from build123d import *

# Parameters (mm, degrees)
SKETCH2_W               = 9.652
SKETCH2_H               = 3.048
SKETCH2_W_2             = 3.048
SKETCH2_H_2             = 35.052
BOSS_EXTRUDE1_DEPTH     = 315
SKETCH3_W               = 25.4
SKETCH3_H               = 76.2
SKETCH3_W_2             = 19.304
SKETCH3_H_2             = 70.104
BOSS_EXTRUDE2_DEPTH     = 50
CUT_EXTRUDE1_DEPTH      = 1
CUT_EXTRUDE1_DEPTH_BACK = 77.2


with BuildPart() as part:
    # Sketch2 → Boss-Extrude1 (new body)
    with BuildSketch(Plane.XY):
        Polygon((-12.7, 0), (-9.652, 0), (-9.652, 35.052), (-9.652, 38.1), (-12.7, 38.1), align=None)
        with Locations((-4.826, 36.576)):
            Rectangle(SKETCH2_W, SKETCH2_H)
        Polygon((0, 38.1), (0, 35.052), (9.652, 35.052), (9.652, 0), (12.7, 0), (12.7, 38.1), align=None)
        with Locations((11.176, -17.526)):
            Rectangle(SKETCH2_W_2, SKETCH2_H_2)
        Polygon((-9.652, -35.052), (-9.652, 0), (-12.7, 0), (-12.7, -38.1), (0, -38.1), (0, -35.052), align=None)
        Polygon((9.652, -35.052), (0, -35.052), (0, -38.1), (12.7, -38.1), (12.7, -35.052), align=None)
    extrude(amount=BOSS_EXTRUDE1_DEPTH)

    # Sketch3 → Boss-Extrude2 (add)
    with BuildSketch(Plane(origin=(0, 0, 0), x_dir=(-1, 0, 0), z_dir=(0, 0, -1))):
        Rectangle(SKETCH3_W, SKETCH3_H)
        Rectangle(SKETCH3_W_2, SKETCH3_H_2, mode=Mode.SUBTRACT)
    extrude(amount=BOSS_EXTRUDE2_DEPTH)

    # Sketch4 → Cut-Extrude1 (cut, two sides)
    with BuildSketch(Plane(origin=(0, 38.1, 0), x_dir=(1, 0, 0), z_dir=(0, 1, 0))) as cut_extrude1_sk:
        Polygon((12.7, 48.301505629), (115.189557491, -14.672106721), (124.098071564, 55.267937569), (-106.281043419, 84.612151011), (-115.189557491, 14.672106721), (-12.7, 1.617644511), (-12.7, 50), (12.7, 50), align=None)
        Polygon((12.7, -1.617644511), (115.189557491, -14.672106721), (12.7, 48.301505629), align=None)
        Polygon((0, 0), (12.7, -1.617644511), (12.7, 48.301505629), (12.534006261, 48.403498707), align=None)
        Polygon((12.534006261, 48.403498707), (12.7, 48.301505629), (12.7, 50), (-12.7, 50), (-12.7, 1.617644511), (0, 0), align=None)
    extrude(amount=CUT_EXTRUDE1_DEPTH, mode=Mode.SUBTRACT)
    extrude(cut_extrude1_sk.sketch, amount=-CUT_EXTRUDE1_DEPTH_BACK, mode=Mode.SUBTRACT)


solid = part.part
Geometry: final body of the model. Coordinates: model frame, mm. A direction names the side the tool comes from. Give positions to 0.01 mm unless a question says otherwise; leave off trailing zeros. Write each loop counter-clockwise with the first axis right and the second up, starting at its lowest first coordinate (ties: lowest second). Pieces come first, ordered by that corner, then holes. Notation, with made-up numbers: (-11, 16) -> (36, 16) arc R23 cw to (36, 47) -> close; hole circle Ø5 at (-25.5, 51.5). An arc over 180 degrees is marked (long way). Answer in a Markdown table with one row per item.
(1) Section query C-C on x = -5.75. Return loops of the section in (y, z), then the cut area to 3 significant figures.
Answers below:
| item | result |
|---|---|
| outline | (-38.1, -0.73) -> (-35.05, -0.73) -> (-35.05, 315) -> (-38.1, 315) -> close; (35.05, -0.73) -> (38.1, -0.73) -> (38.1, 315) -> (35.05, 315) -> close |
| area | 1,920 mm^2 |
(2) Draft query along X for faces 3 (the flat face through (9.652, 0, 160)), 4 (the flat face through (0, 35.052, 159)), 5 (the flat face through (-10, 3, 315)), 6 (the flat face through (-10.407, 3, -1.326)). Return one class per face: +X half, -X half, draft (parallel to the pull), parting line (faces both ways), or undercut.
Answers below:
| item | result |
|---|---|
| face 3 | undercut |
| face 4 | undercut |
| face 5 | draft |
| face 6 | +X half |
(3) Ray query, line 1 along X through (y, z) = (-2, 140.5); line 2 along Y through (x, z) = (4.5, 220); line 3 along Z through (x, y) = (11.25, -10). Return the intervals inside material, ascending. Write a range as [from, to].
Answers below:
| item | result |
|---|---|
| line 1 | [-12.7, -9.65], [9.65, 12.7] |
| line 2 | [-38.1, -35.05], [35.05, 38.1] |
| line 3 | [1.43, 315] |
(4) Set-up query: faces 1 (the flat face through (12.7, -1, 161)), 2 (the flat face through (-9.652, 0, 159)). Return all of +Z, -Z, +X, -X, +Y, -Y with unobstructed straight access to the full face (end or side cutting, diameter ignored); none if empty.
Answers below:
| item | result |
|---|---|
| face 1 | +Z, -Z, +X, +Y, -Y |
| face 2 | +Z, -Z |
(5) Pin query (flat end, axial travel): pin 1 (8 mm diameter, centred on x = 9, y = 7.5, fed in from +Z). Return the tip coordinate at first contact, or that it passes through.
Answers below:
| item | result |
|---|---|
| pin 1 | z = 315 |
(6) Section query B-B on z = 54. Return loops of the section in (x, y).
Answers below:
| item | result |
|---|---|
| outline | (-12.7, -38.1) -> (12.7, -38.1) -> (12.7, 38.1) -> (-12.7, 38.1) -> close; hole (-9.65, -35.05) -> (9.65, -35.05) -> (9.65, 35.05) -> (-9.65, 35.05) -> close |
(7) Section query A-A on y = -28.5. Return loops of the section in (x, z), then the cut area to 3 significant figures.
Answers below:
| item | result |
|---|---|
| outline | (-12.7, -1.62) -> (-9.65, -1.23) -> (-9.65, 315) -> (-12.7, 315) -> close; (9.65, 1.23) -> (12.7, 1.62) -> (12.7, 315) -> (9.65, 315) -> close |
| area | 1,920 mm^2 |
